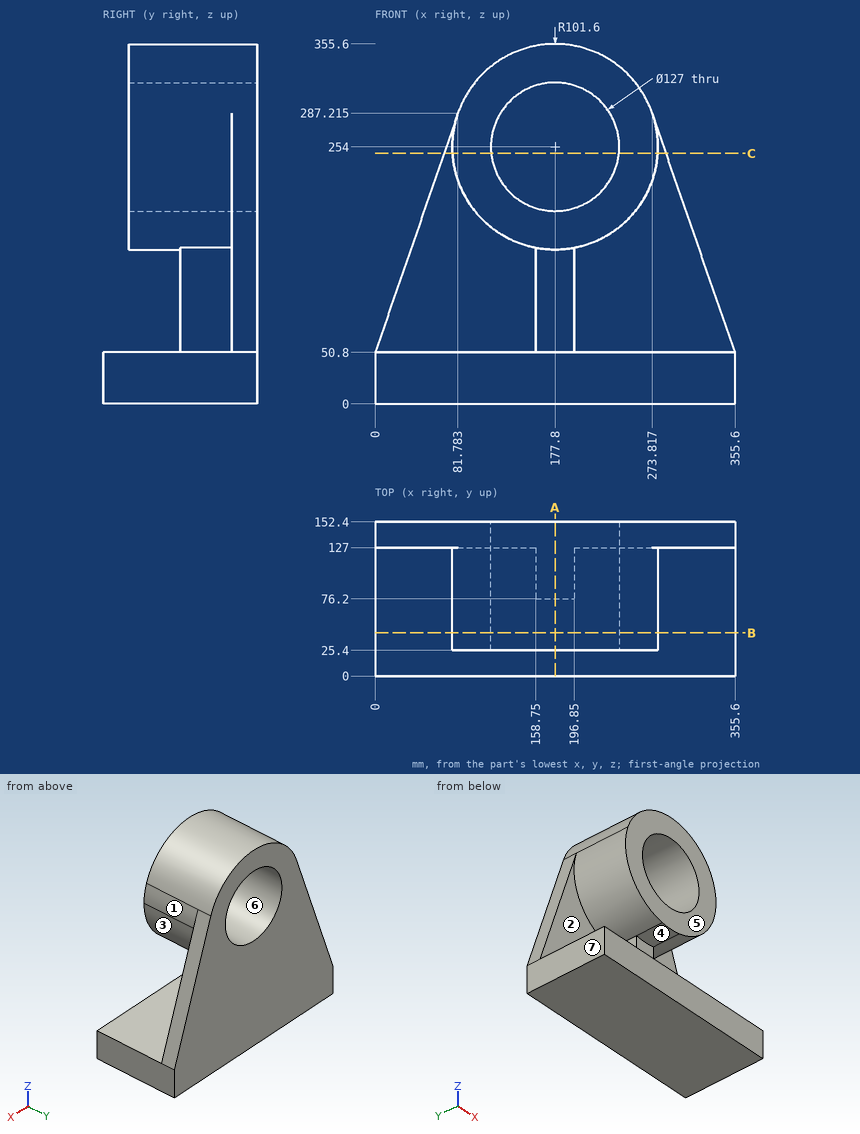
Job drawing, mm, ordinate dimensions from the low corner. One solid piece. A direction names the side the tool comes from. Coordinates: 2 decimals unless noted, no trailing zeros. Order: outer loops, then holes, each group sorted by start corner. A loop starts at its lowest first (then second) coordinate and runs counter-clockwise, first axis right, second up. Notation, with made-up numbers: (46.5, 5) -> (103.5, 5) arc R22 cw to (103.5, 29) -> close; hole circle Ø4 at (-5.75, 66). An arc over 180 degrees is marked (long way). Put each result on its own line as item: value. Start each with the question number.
(1) Pin check, flat tips, straight feed: pin 1 Ø15 at (y, z) = (97, 80) entering from +X; pin 2 Ø12 at (y, z) = (47, 277) entering from -X; pin 3 Ø12 at (y, z) = (98.5, 314) entering from +X. Stop position of each tip, or through.
(2) Mould opens along X. For the marked faces 5, 6 and 7 say: pulls with the +X half, pulls with the -X half, needs draft (parallel to the pull), parting line crosses it, or undercut.
(3) Probe line 1 along Z through (x, y) = (177, 80) (1 decimal); line 2 along Z through (x, y) = (154.5, 97); line 3 along Y through (x, z) = (250.5, 279.5). List the from-to ranges inside material, lowest first. Write a range as [from, to].
(4) Which spindle directions (+Z, -Z, +X, -X, +Y, -Y) get a long thin tool onto all of the face, cutting with end or side? Do the marked faces 1, 2, 3 and 4. Say none if no direction does.
(5) Band-saw the part on C-C (z = 247.5). Give the cut face in (x, y).
(6) Band-saw the part on A-A (x = 177.8). Give the cut face in (y, z), then the cut area to 3 significant figures.
(7) Band-saw the part on B-B (y = 42.5). Count the separate pieces of the cut face and the enclosed holes in it, then the cut area to 3 significant figures.
Determined:
1. pin 1: stops at x = 196.85
1. pin 2: stops at x = 77.63
1. pin 3: stops at x = 263.86
2. face 5: needs draft
2. face 6: undercut
2. face 7: pulls with the -X half
3. line 1: z = [0, 190.5], [317.5, 355.6]
3. line 2: z = [0, 50.8], [155.11, 194.93], [313.07, 352.89]
3. line 3: y = [25.4, 152.4]
4. face 1: +Z, +X, -Y
4. face 2: -X, -Y
4. face 3: +X, -Y
4. face 4: -Y
5. outline: (68.04, 127) -> (76.41, 127) -> (76.41, 25.4) -> (114.63, 25.4) -> (114.63, 152.4) -> (68.04, 152.4) -> close; (240.97, 25.4) -> (279.19, 25.4) -> (279.19, 127) -> (287.56, 127) -> (287.56, 152.4) -> (240.97, 152.4) -> close
6. outline: (0, 0) -> (152.4, 0) -> (152.4, 190.5) -> (25.4, 190.5) -> (25.4, 152.4) -> (76.2, 152.4) -> (76.2, 50.8) -> (0, 50.8) -> close; (25.4, 317.5) -> (152.4, 317.5) -> (152.4, 355.6) -> (25.4, 355.6) -> close
6. area: 25,200 mm²
7. separate pieces: 2
7. enclosed holes: 1
7. area: 37,800 mm²
